from build123d import *

# Parameters (mm, degrees)
SKETCH_1_W      = 28
SKETCH_1_H      = 54
SKETCH_1_R      = 1.5
SKETCH_1_W_2    = 24
SKETCH_1_H_2    = 42
EXTRUDE_1_DEPTH = 2
SKETCH_2_W      = 20
SKETCH_2_H      = 54
SKETCH_2_R      = 2
EXTRUDE_2_DEPTH = 1.5
FILLET_1_R      = 8


with BuildPart() as part:
    # 草图1 → 凸台-拉伸1 (new body)
    with BuildSketch(Plane(origin=(0, 0, 0), x_dir=(0, 0, -1), z_dir=(1, 0, 0))):
        with Locations((-14, 27)):
            Rectangle(SKETCH_1_W, SKETCH_1_H)
        with Locations((-7.5, 51)):
            Circle(SKETCH_1_R, mode=Mode.SUBTRACT)
        with Locations((-17.5, 51)):
            Circle(SKETCH_1_R, mode=Mode.SUBTRACT)
        with Locations(Location((-7.5, 3, 0), (0, 0, 180))):
            Circle(SKETCH_1_R, mode=Mode.SUBTRACT)
        with Locations(Location((-17.5, 3, 0), (0, 0, 180))):
            Circle(SKETCH_1_R, mode=Mode.SUBTRACT)
        with Locations((-13, 27)):
            Rectangle(SKETCH_1_W_2, SKETCH_1_H_2, mode=Mode.SUBTRACT)
    extrude(amount=EXTRUDE_1_DEPTH)

    # 草图2 → 凸台-拉伸2 (add)
    with BuildSketch(Plane(origin=(0, 0, 0), x_dir=(-1, 0, 0), z_dir=(0, 0, -1))):
        with Locations((-10, 27)):
            Rectangle(SKETCH_2_W, SKETCH_2_H)
        with Locations(Location((-16, 4, 0), (0, 0, 90))):
            Circle(SKETCH_2_R, mode=Mode.SUBTRACT)
        with Locations((-4, 4)):
            Circle(SKETCH_2_R, mode=Mode.SUBTRACT)
        with Locations(Location((-4, 19, 0), (0, 0, 270))):
            Circle(SKETCH_2_R, mode=Mode.SUBTRACT)
        with Locations(Location((-16, 19, 0), (0, 0, 270))):
            Circle(SKETCH_2_R, mode=Mode.SUBTRACT)
    extrude(amount=EXTRUDE_2_DEPTH)

    # 圆角1
    fillet_1_edges = [part.edges().sort_by_distance(p)[0] for p in [
        (1, 54, 28),
    ]]
    fillet(fillet_1_edges, radius=FILLET_1_R)


solid = part.part
Input: part model. Units: mm. Frame: model coordinates. A direction names the side the tool comes from. Give positions to 0.01 mm unless a question says otherwise; leave off trailing zeros. Loops run counter-clockwise (first coordinate to the right, second up) from the corner with the lowest first, then second, coordinate; pieces in that order, holes last. Notation, with made-up numbers: (-27.5, -12) -> (-1.5, -12) arc R20 ccw to (-1.5, 17) -> close; hole circle Ø2 at (-22, 23.5). An arc over 180 degrees is marked (long way). Answer as a JSON object with one key per item and string values. Group by question number.
Item 1: Pull-direction query (Z, two-part tool) for faces 4 (the flat face through (1, 54, 5)), 5 (the cylindrical face through (0.99, 1.99, 6.39)), 6 (the flat face through (1, 23, 28)), 7 (the cylindrical face through (0.986, 49.536, 7.825)); classes: released by +Z, released by -Z, zero draft, split by the parting line, or undercut.
Item 2: Cut plane C-C, the plane x = 16. Return the cut outline in (y, z), and give its area (3 significant figures).
Item 3: Pin query (flat end, axial travel): P1, Ø3.5, axis at y = 3, z = 7.5, coming from the -X side; P2, Ø10, axis at y = 10, z = 8, coming from the +X side; P3, Ø2.5, axis at y = 3, z = 17.5, coming from the -X side; P4, Ø5, axis at x = 8.5, y = 30.5, coming from the +Z side. Return the tip coordinate at first contact, or that it passes through.
Item 4: Reachability of faces 1 (the flat face through (1, 6, 13)), 2 (the cylindrical face through (5.6, 2.8, -0.7)), 3 (the flat face through (11, 27, 0)) from +Z, -Z, +X, -X, +Y, -Y: full face, straight path, thin tool, end or side. Return the list, or none.
Item 5: Cut plane D-D, the plane y = 27. Return the cut outline in (x, z), and give its area (3 significant figures).
Item 6: Cut plane B-B, the plane z = 12.5. Return the cut outline in (x, y).
Item 7: Line query: probe 1 along X at (y, z) = (19, -0.7); probe 2 along Y at (x, z) = (0.5, 7.5); probe 3 along Z at (x, y) = (1, 13). Output: solid intervals per line, ascending.
Item 8: Cut plane A-A, the plane z = 7.5. Return the cut outline in (x, y), and give its area (3 significant figures).
Checks:
{
 "1": {"face 4": "zero draft", "face 5": "undercut", "face 6": "released by +Z", "face 7": "undercut"},
 "2": {"outline": "(0, -1.5) -> (2, -1.5) -> (2, 0) -> (0, 0) -> close; (6, -1.5) -> (17, -1.5) -> (17, 0) -> (6, 0) -> close; (21, -1.5) -> (54, -1.5) -> (54, 0) -> (21, 0) -> close", "area": "69.0 mm²"},
 "3": {"P1": "stops at x = 0", "P2": "stops at x = 2", "P3": "passes through", "P4": "stops at z = 0"},
 "4": {"face 1": "+X, -X", "face 2": "+Z, -Z", "face 3": "+Z, +X, +Y, -Y"},
 "5": {"outline": "(0, -1.5) -> (20, -1.5) -> (20, 0) -> (2, 0) -> (2, 1) -> (0, 1) -> close; (0, 25) -> (2, 25) -> (2, 28) -> (0, 28) -> close", "area": "38.0 mm²"},
 "6": {"outline": "(0, 0) -> (2, 0) -> (2, 6) -> (0, 6) -> close; (0, 48) -> (2, 48) -> (2, 54) -> (0, 54) -> close"},
 "7": {"probe 1": "x = 0 to 2, 6 to 14, 18 to 20", "probe 2": "y = 0 to 1.5, 4.5 to 6, 48 to 49.5, 52.5 to 54", "probe 3": "z = -1.5 to 1, 25 to 28"},
 "8": {"outline": "(0, 0) -> (2, 0) -> (2, 1.5) -> (0, 1.5) -> close; (0, 4.5) -> (2, 4.5) -> (2, 6) -> (0, 6) -> close; (0, 48) -> (2, 48) -> (2, 49.5) -> (0, 49.5) -> close; (0, 52.5) -> (2, 52.5) -> (2, 54) -> (0, 54) -> close", "area": "12.0 mm²"}
}
